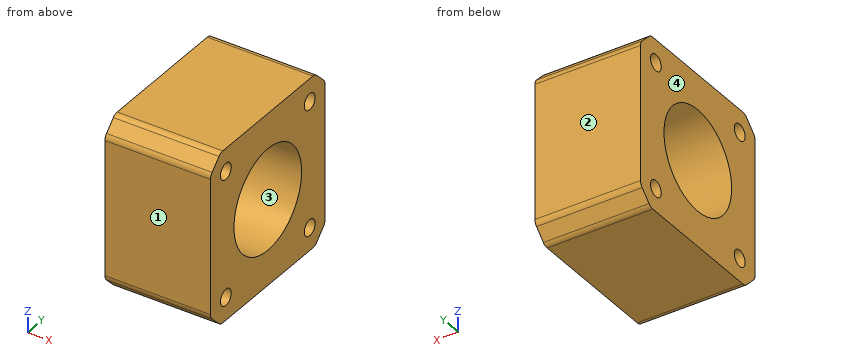
from build123d import *

# Parameters (mm, degrees)
BOSS_EXTRUDE1_DEPTH     = 26
FILLET1_R               = 2
SKETCH2_R               = 12.5
CUT_EXTRUDE1_DEPTH      = 27
SKETCH3_R               = 2
CUT_EXTRUDE2_DEPTH      = 27
LPATTERN1_COUNT         = 2
LPATTERN1_PITCH         = 31
MIRROR1_COPY_1_SKETCH_R = 2
MIRROR1_COPY_1_DEPTH    = 27


with BuildPart() as part:
    # Sketch1 → Boss-Extrude1 (new body)
    with BuildSketch(Plane(origin=(0, 0, 0), x_dir=(0, 0, -1), z_dir=(1, 0, 0))):
        Polygon((-21.15, 17.458030253), (-17.458030253, 21.15), (17.458030253, 21.15), (21.15, 17.458030253), (21.15, -17.458030253), (17.458030253, -21.15), (-17.458030253, -21.15), (-21.15, -17.458030253), align=None)
    extrude(amount=BOSS_EXTRUDE1_DEPTH)

    # Fillet1
    fillet1_edges = [part.edges().sort_by_distance(p)[0] for p in [
        (13, 17.458030253, 21.15),
        (13, 21.15, 17.458030253),
        (13, 21.15, -17.458030253),
        (13, 17.458030253, -21.15),
        (13, -17.458030253, -21.15),
        (13, -21.15, -17.458030253),
        (13, -21.15, 17.458030253),
        (13, -17.458030253, 21.15),
    ]]
    fillet(fillet1_edges, radius=FILLET1_R)

    # Sketch2 → Cut-Extrude1 (cut, through all)
    with BuildSketch(Plane(origin=(26, 0, 0), x_dir=(0, 0, -1), z_dir=(1, 0, 0))):
        Circle(SKETCH2_R)
    extrude(amount=-CUT_EXTRUDE1_DEPTH, mode=Mode.SUBTRACT)

    # Sketch3 → Cut-Extrude2 (cut, through all)
    with BuildSketch(Plane(origin=(26, 0, 0), x_dir=(0, 0, -1), z_dir=(1, 0, 0))):
        with Locations((-15.5, 15.5)):
            Circle(SKETCH3_R)
    cut_extrude2 = extrude(amount=-CUT_EXTRUDE2_DEPTH, mode=Mode.SUBTRACT)

    # LPattern1: Cut-Extrude2 ×2
    with Locations(*[(0, 0, -i * LPATTERN1_PITCH) for i in range(1, LPATTERN1_COUNT)]):
        add(cut_extrude2, mode=Mode.SUBTRACT)

    # Mirror1: Cut-Extrude2 across plane
    add(cut_extrude2.mirror(Plane.ZX), mode=Mode.SUBTRACT)

    # Mirror1 copy 1 sketch → Mirror1 copy 1 (cut, through all)
    with BuildSketch(Plane(origin=(26, 0, -31), x_dir=(0, 0, -1), z_dir=(1, 0, 0))):
        with Locations((-15.5, -15.5)):
            Circle(MIRROR1_COPY_1_SKETCH_R)
    extrude(amount=-MIRROR1_COPY_1_DEPTH, mode=Mode.SUBTRACT)


solid = part.part
Verification items for the finished model (mm, model axes). Face numbers are marked on the shaded views. Round coordinates to 2 decimals unless told otherwise and drop trailing zeros. Order: outer loops, then holes, each group sorted by start corner. A loop starts at its lowest first (then second) coordinate and runs counter-clockwise, first axis right, second up.
1. Section check C-C on y = -15.5. Record the cut outline in (x, z).
Final values:
outline: (0, -21.15) - (26, -21.15) - (26, -17.5) - (0, -17.5) - close; (0, -13.5) - (26, -13.5) - (26, 13.5) - (0, 13.5) - close; (0, 17.5) - (26, 17.5) - (26, 21.15) - (0, 21.15) - close
2. Section check A-A on y = 0. Record the cut outline in (x, z), then the cut area to 3 significant figures.
Final values:
outline: (0, -21.15) - (26, -21.15) - (26, -12.5) - (0, -12.5) - close; (0, 12.5) - (26, 12.5) - (26, 21.15) - (0, 21.15) - close
area: 450 mm2
3. Release check for a two-part mould opening along Y. For the marked faces 1, 2, 3 and 4 record: +Y half, -Y half, draft (parallel to the pull), parting line (faces both ways), or undercut.
Final values:
face 1: -Y half
face 2: +Y half
face 3: undercut
face 4: draft
4. Go/stop test with a flat-tipped pin: P1, Ø1, axis at y = -7.5, z = 8.5, coming from the +X side. Record where the tip stops, or that it passes through.
Final values:
P1: passes through
5. Thickness scan on L1, parallel to Y at x = 6.25, z = 15.5; L2, parallel to Z at x = 7.5, y = -6; L3, parallel to Y at x = 11, z = -2.5. Record the ranges inside material, lowest first.
Final values:
L1: y = -21.15 to -17.5, -13.5 to 13.5, 17.5 to 21.15
L2: z = -21.15 to -10.97, 10.97 to 21.15
L3: y = -21.15 to -12.25, 12.25 to 21.15
6. Section check D-D on x = 13. Record the cut outline in (y, z), then the cut area to 3 significant figures.
Final values:
outline: (-21.15, -16.63) arc R2 ccw to (-20.56, -18.04) - (-18.04, -20.56) arc R2 ccw to (-16.63, -21.15) - (16.63, -21.15) arc R2 ccw to (18.04, -20.56) - (20.56, -18.04) arc R2 ccw to (21.15, -16.63) - (21.15, 16.63) arc R2 ccw to (20.56, 18.04) - (18.04, 20.56) arc R2 ccw to (16.63, 21.15) - (-16.63, 21.15) arc R2 ccw to (-18.04, 20.56) - (-20.56, 18.04) arc R2 ccw to (-21.15, 16.63) - close; hole circle Ø4 at (-15.5, -15.5); hole circle Ø4 at (-15.5, 15.5); hole circle Ø25 at (0, 0); hole circle Ø4 at (15.5, -15.5); hole circle Ø4 at (15.5, 15.5)
area: 1,220 mm2
7. Section check B-B on z = 10. Record the cut outline in (x, y).
Final values:
outline: (0, -21.15) - (26, -21.15) - (26, -7.5) - (0, -7.5) - close; (0, 7.5) - (26, 7.5) - (26, 21.15) - (0, 21.15) - close
